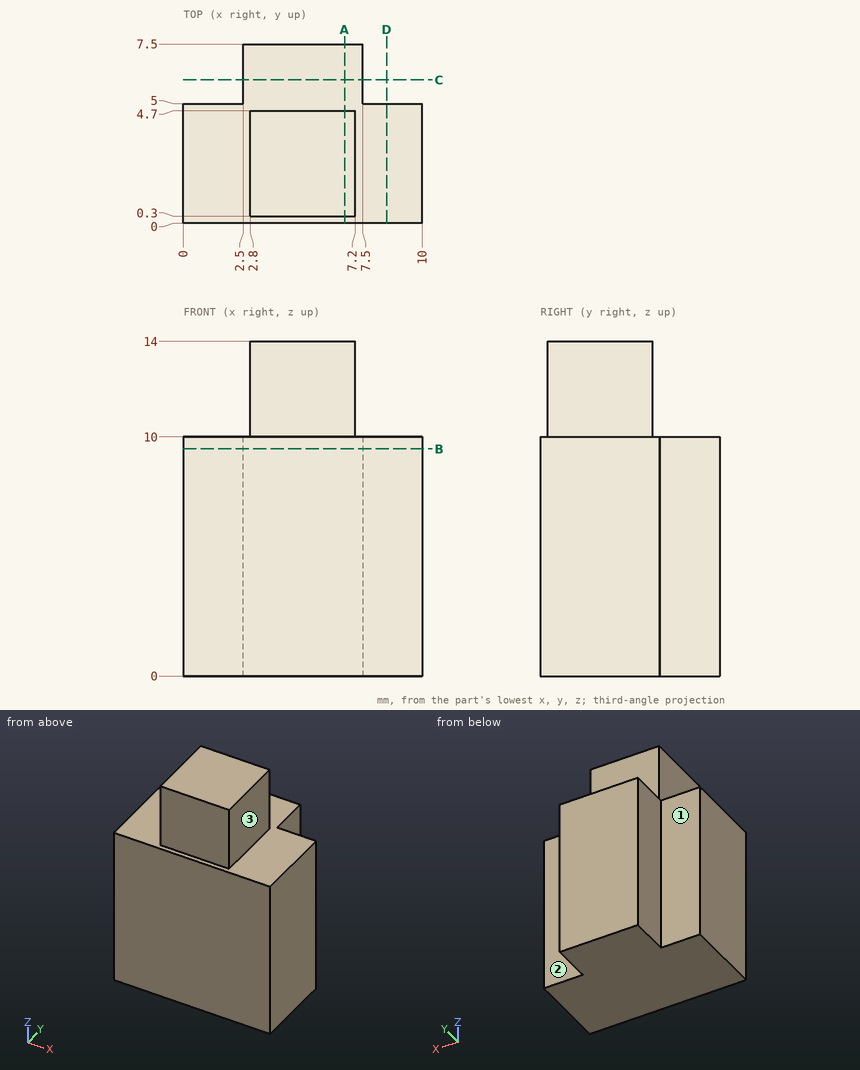
For this review, use the dimensioned drawing (mm, ordinates from the lowest corner) and the shaded views. A direction names the side the tool comes from. Round coordinates to 2 decimals unless told otherwise and drop trailing zeros. Loops run counter-clockwise (first coordinate to the right, second up) from the corner with the lowest first, then second, coordinate; pieces in that order, holes last. Notation, with made-up numbers: M 73.5,-39.75 L 83.5,-39.75 A20 cw 83.5,-0.75 Z; hole C 56.25,89.5 d7. An arc over 180 degrees is marked long. Answer as CSV lines item,"result".
1. To check wall thickness, follow L1, parallel to X at y = 2.25, z = 11.25; L2, parallel to Z at x = 5.5, y = 6.75; L3, parallel to X at y = 6, z = 9.25. State the ranges of each line that lie inside material, in increasing order. Write a range as [from, to].
Outcome:
L1,"x = [2.8, 7.2]"
L2,"z = [0, 10]"
L3,"x = [2.5, 7.5]"
2. We need section A-A (x = 6.75). Give the boundary of the cut face in (y, z), plus the area to 3 significant figures.
Outcome:
outline,"M 0,0 L 7.5,0 L 7.5,10 L 4.7,10 L 4.7,14 L 0.3,14 L 0.3,10 L 0,10 Z"
area,"92.6 mm2"
3. For the marked faces 1, 2 and 3, list the 3-axis set-ups (+Z, -Z, +X, -X, +Y, -Y) from which the entire face can be reached by the end or side of a thin tool; tool diameter is ignored.
Outcome:
face 1,"+Z, -Z, -X, +Y"
face 2,"+Z, -Z, +X, +Y"
face 3,"+Z, +X, +Y, -Y"
4. We need section B-B (z = 9.5). Give the boundary of the cut face in (x, y), plus the area to 3 significant figures.
Outcome:
outline,"M 0,0 L 10,0 L 10,5 L 7.5,5 L 7.5,7.5 L 2.5,7.5 L 2.5,5 L 0,5 Z"
area,"62.5 mm2"
5. We need section D-D (x = 8.5). Give the boundary of the cut face in (y, z), plus the area to 3 significant figures.
Outcome:
outline,"M 0,0 L 5,0 L 5,10 L 0,10 Z"
area,"50.0 mm2"
6. Insertion check: pin 1 Ø1.2 at (x, z) = (4, 13) entering from +Y; pin 2 Ø4.5 at (x, z) = (5, 13) entering from -Y; pin 3 Ø1.5 at (x, y) = (1.5, 2.5) entering from +Z. Each pin has a flat end and moves straight along its axis. Give the tip position at first contact, or say it passes through.
Outcome:
pin 1,"stops at y = 4.7"
pin 2,"stops at y = 0.3"
pin 3,"stops at z = 10"
7. We need section C-C (y = 6). Give the boundary of the cut face in (x, z), plus the area to 3 significant figures.
Outcome:
outline,"M 2.5,0 L 7.5,0 L 7.5,10 L 2.5,10 Z"
area,"50.0 mm2"
